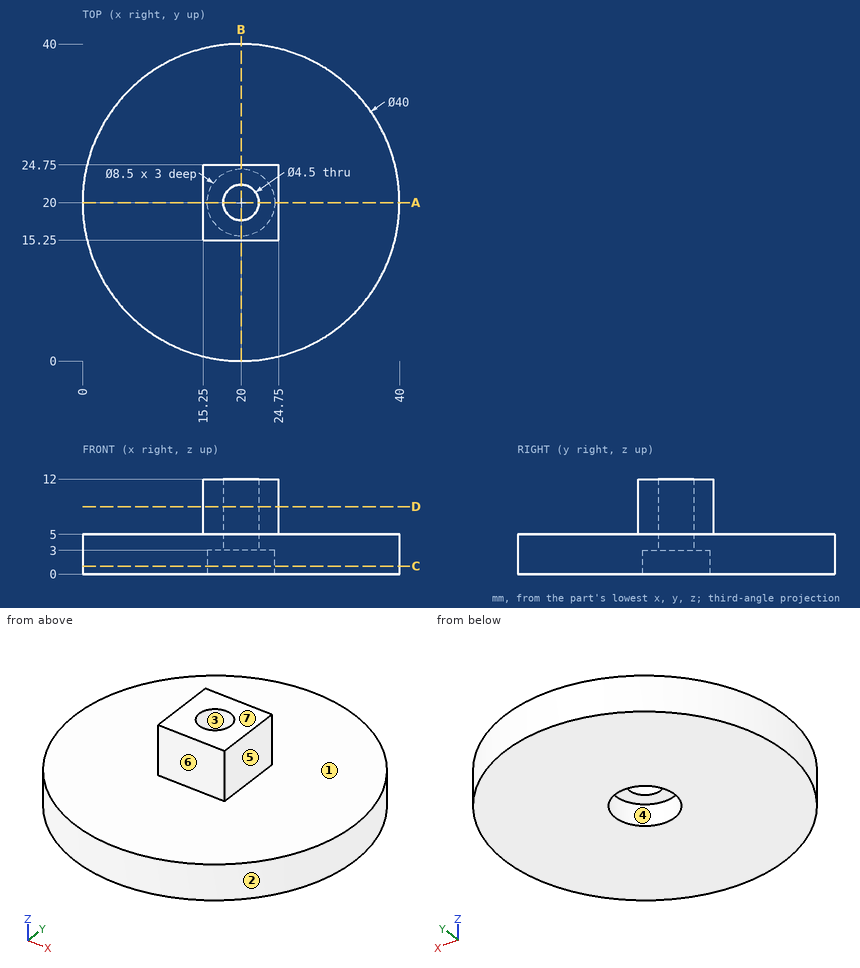
Geometry: see drawing. Coordinates: mm, zero at the bounding-box minimum. A direction names the side the tool comes from. Round coordinates to 2 decimals unless told otherwise and drop trailing zeros. Loops run counter-clockwise (first coordinate to the right, second up) from the corner with the lowest first, then second, coordinate; pieces in that order, holes last.
(1) Contact query for flat-ended pins moving along their axis: pin 1 Ø5 at (x, z) = (5, 9) entering from +Y; pin 2 Ø2 at (x, z) = (29, 3) entering from +Y; pin 3 Ø5.5 at (x, z) = (18.5, 8.5) entering from -Y; pin 4 Ø2 at (y, z) = (32, 3) entering from +X. Output: stop coordinate, or through.
From the geometry:
pin 1: passes through
pin 2: stops at y = 38.33
pin 3: stops at y = 15.25
pin 4: stops at x = 36.7
(2) Section query A-A (y = 20). Output: boundary loops of the cut face in (x, z).
From the geometry:
outline: (0, 0) - (15.75, 0) - (15.75, 3) - (17.75, 3) - (17.75, 12) - (15.25, 12) - (15.25, 5) - (0, 5) - close; (22.25, 3) - (24.25, 3) - (24.25, 0) - (40, 0) - (40, 5) - (24.75, 5) - (24.75, 12) - (22.25, 12) - close
(3) Access query for the marked faces 4, 5, 6 and 7. Directions: +Z, -Z, +X, -X, +Y, -Y. A direction counts if a zero-diameter tool reaches every point of the face in a straight line with its end or side. Return the directions, or none.
From the geometry:
face 4: -Z
face 5: +Z, +X, +Y, -Y
face 6: +Z, +X, -X, -Y
face 7: +Z, +X, -X, +Y, -Y
(4) Pull-direction query (X, two-part tool) for the marked faces 1, 2 and 3; classes: +X half, -X half, draft (parallel to the pull), parting line (faces both ways), or undercut.
From the geometry:
face 1: draft
face 2: parting line
face 3: undercut
(5) Section query C-C (z = 1). Output: boundary loops of the cut face in (x, y).
From the geometry:
outline: circle Ø40 at (20, 20); hole circle Ø8.5 at (20, 20)
(6) Section query D-D (z = 8.5). Output: boundary loops of the cut face in (x, y), and give its area (3 significant figures).
From the geometry:
outline: (15.25, 15.25) - (24.75, 15.25) - (24.75, 24.75) - (15.25, 24.75) - close; hole circle Ø4.5 at (20, 20)
area: 74.3 mm2
(7) Material intervals for probe 1 along X at (y, z) = (20, 6); probe 2 along Z at (x, y) = (9, 22), sorted ascending.
From the geometry:
probe 1: x = 15.25 to 17.75, 22.25 to 24.75
probe 2: z = 0 to 5
